```python
from build123d import *

# Parameters (mm, degrees)
ESQUISSE1_W                  = 40
ESQUISSE1_H                  = 40
ESQUISSE1_R                  = 1.5
BOSS_EXTRU_1_DEPTH           = 10
ENL_V_MAT_EXTRU_1_DEPTH      = 31
R_P_TITION_CIRCULAIRE1_COUNT = 7


with BuildPart() as part:
    # Esquisse1 → Boss.-Extru.1 (new body)
    with BuildSketch(Plane.XY):
        Rectangle(ESQUISSE1_W, ESQUISSE1_H)
        with Locations((-16, 16)):
            Circle(ESQUISSE1_R, mode=Mode.SUBTRACT)
        with Locations(Location((16, 16, 0), (0, 0, 180))):
            Circle(ESQUISSE1_R, mode=Mode.SUBTRACT)
        with Locations((16, -16)):
            Circle(ESQUISSE1_R, mode=Mode.SUBTRACT)
        with Locations(Location((-16, -16, 0), (0, 0, 180))):
            Circle(ESQUISSE1_R, mode=Mode.SUBTRACT)
    extrude(amount=BOSS_EXTRU_1_DEPTH)

    # Esquisse2 → Enlèv. mat.-Extru.1 (cut, through all)
    with BuildSketch(Plane.XY.offset(10)):
        with BuildLine():
            ThreePointArc((4.013801979, 6.335565774), (2.093936315, 7.201765805), (0.00893123, 7.499994682))
            ThreePointArc((0.00893123, 7.499994682), (1.579824901, 13.460592117), (5.558485397, 18.168743492))
            ThreePointArc((5.558485397, 18.168743492), (6.684148303, 17.785448026), (7.783629485, 17.332487186))
            ThreePointArc((7.783629485, 17.332487186), (4.864634522, 12.188517309), (4.013801979, 6.335565774))
        make_face()
    enl_v_mat_extru_1 = extrude(amount=-ENL_V_MAT_EXTRU_1_DEPTH, mode=Mode.SUBTRACT)

    # Répétition circulaire1: Enlèv. mat.-Extru.1 ×7 about axis
    r_p_tition_circulaire1_axis = Axis((0, 0, 0), (0, 0, 1))
    for i in range(1, R_P_TITION_CIRCULAIRE1_COUNT):
        add(enl_v_mat_extru_1.rotate(r_p_tition_circulaire1_axis, i * 360 / R_P_TITION_CIRCULAIRE1_COUNT), mode=Mode.SUBTRACT)

    # Esquisse3 → Enlèvement de matière-Révolution1 (revolve, cut)
    with BuildSketch(Plane(origin=(0, 0, 0), x_dir=(0, 0, -1), z_dir=(1, 0, 0))):
        with BuildLine():
            Line((0, 19), (0, 7.5))
            ThreePointArc((0, 7.5), (-0.844387246, 13.25), (0, 19))
        make_face()
        with BuildLine():
            Line((-10, 19), (-10, 7.5))
            ThreePointArc((-10, 7.5), (-9.155612754, 13.25), (-10, 19))
        make_face()
    revolve(axis=Axis((0, 0, -0.5), (0, 0, 1)), mode=Mode.SUBTRACT)


solid = part.part
```
Work out the finished part from the listing and answer in its coordinate system (mm). A direction names the side the tool comes from. Round coordinates to 2 decimals unless told otherwise and drop trailing zeros.
(1) Find the intervals of material crossed by L1, parallel to Y at x = 16, z = 5.25; L2, parallel to X at y = -6.5, z = 1.5; L3, parallel to Y at x = 8.5, z = 5.5, in increasing order.
Computed values:
L1: y = -20 to -17.5, -14.5 to -10.25, -8.5 to 4.61, 7.3 to 14.5, 17.5 to 20
L2: x = -20 to -7.74, -3.74 to 9.02, 14.67 to 20
L3: y = -20 to -6.28, -2.05 to 1.64, 6.21 to 20
(2) Each of these flat-tipped pins is pushed along its axis until it touches: P1, Ø2, axis at x = 13, y = -1.5, coming from the +Z side; P2, Ø2.5, axis at x = 16, y = 16, coming from the -Z side. Where does it stop, or does it pass through?
Computed values:
P1: stops at z = 9.19
P2: passes through
(3) For faces 1 (the flat face through (0, 0, 0)), 2 (the cylindrical face through (11.42, 7.14, 5.07)), determine the directions among +Z, -Z, +X, -X, +Y, -Y from which every point of the face is accessible in a straight line to the end or side of a thin tool.
Computed values:
face 1: -Z, +X, -X, +Y, -Y
face 2: +Z, -Z
(4) The part is cut by section A-A, the plane x = -15. Give the number of separate pieces and of enclosed holes in the cut face, and give its area (3 significant figures).
Computed values:
separate pieces: 4
enclosed holes: 0
area: 301 mm2
(5) The mould has two halves that part along X. Classify faces 3 (the flat face through (-8, -18, 10)), 4 (the flat face through (-20, 0, 5)), 5 (the cylindrical face through (-18.83, 2.54, 5.07)): pulls with the +X half, pulls with the -X half, needs draft (parallel to the pull), parting line crosses it, or undercut.
Computed values:
face 3: needs draft
face 4: pulls with the -X half
face 5: undercut
